from build123d import *

# Parameters (mm, degrees)
BOSS_EXTRUDE1_DEPTH      = 15.06
BOSS_EXTRUDE2_DEPTH      = 3.175
SKETCH7_W                = 15.06
SKETCH7_H                = 28.575
BOSS_EXTRUDE3_DEPTH      = 25.4
BOSS_EXTRUDE3_DEPTH_BACK = 2.54
CUT_EXTRUDE1_START       = -0.254
CUT_EXTRUDE1_DEPTH       = 14.552
BOSS_EXTRUDE4_DEPTH      = 8.1
SKETCH8_R                = 5.1
CUT_EXTRUDE3_DEPTH       = 826.597233992
SKETCH15_R               = 6.096
CUT_EXTRUDE4_DEPTH       = 823.185140665
CUT_EXTRUDE6_DEPTH       = 0.254
SKETCH22_W               = 12.7
SKETCH22_H               = 3
CUT_EXTRUDE8_DEPTH       = 2.5
BOSS_EXTRUDE5_START      = -3.175
SKETCH23_R               = 1.13
BOSS_EXTRUDE5_DEPTH      = 11.377
CUT_EXTRUDE9_DEPTH       = 2
SKETCH25_W               = 12.7
SKETCH25_H               = 2.5
BOSS_EXTRUDE6_DEPTH      = 2
CUT_EXTRUDE11_DEPTH      = 826.590147754
BOSS_EXTRUDE7_DEPTH      = 19.886
FILLET1_R                = 2
SKETCH31_R               = 2
CUT_EXTRUDE12_DEPTH      = 826.405127723


with BuildPart() as part:
    # Sketch1 → Boss-Extrude1 (new body)
    with BuildSketch(Plane.XY):
        with BuildLine():
            ThreePointArc((768.898502001, 253.220496825), (772.473384001, 257.975032047), (771.279316377, 263.802517698))
            Line((771.279316377, 263.802517698), (754.541770866, 286.976250421))
            ThreePointArc((754.541770866, 286.976250421), (750.425558167, 289.761469174), (745.483441324, 289.235986934))
            Line((745.483441324, 289.235986934), (736.959388492, 285.051606769))
            Line((736.959388492, 285.051606769), (732.179744734, 283.489883627))
            ThreePointArc((732.179744734, 283.489883627), (729.115297933, 279.264699802), (732.179762843, 275.03952911))
            Line((732.179762843, 275.03952911), (736.959413295, 273.477826454))
            ThreePointArc((736.959413295, 273.477826454), (738.543478356, 272.323947498), (739.148316802, 270.459847389))
            Line((739.148316802, 270.459847389), (741.478441562, 249.420712606))
            ThreePointArc((741.478441562, 249.420712606), (746.159744473, 243.429023652), (753.614349117, 244.926956583))
            ThreePointArc((753.614349117, 244.926956583), (754.705448313, 245.901255726), (755.838945539, 246.825885552))
            Line((755.838945539, 246.825885552), (768.898502001, 253.220496825))
        make_face()
    extrude(amount=BOSS_EXTRUDE1_DEPTH)

    # Sketch1<4> → Boss-Extrude2 (add)
    with BuildSketch(Plane.XY):
        with BuildLine():
            Line((767.984780823, 261.422994326), (751.247235317, 284.596727042))
            ThreePointArc((751.247235317, 284.596727042), (747.696485062, 285.758701464), (745.498379419, 282.7377176))
            Line((745.498379419, 282.7377176), (745.498449109, 250.217566764))
            ThreePointArc((745.498449109, 250.217566764), (747.408500645, 247.30543855), (750.840510516, 247.897127523))
            ThreePointArc((750.840510516, 247.897127523), (758.022031433, 253.136086658), (766.249615232, 256.501766428))
            ThreePointArc((766.249615232, 256.501766428), (768.405251042, 258.508228422), (767.984780823, 261.422994326))
        make_face()
    extrude(amount=-BOSS_EXTRUDE2_DEPTH)

    # Sketch7 → Boss-Extrude3 (add, two sides)
    with BuildSketch(Plane(origin=(759.782778814, 84.147408332, 0), x_dir=(0, 0, 1), z_dir=(-0.9939228549686344, -0.11007887340901991, 0))) as boss_extrude3_sk:
        with Locations((7.53, 176.895767228)):
            Rectangle(SKETCH7_W, SKETCH7_H)
    extrude(amount=BOSS_EXTRUDE3_DEPTH)
    extrude(boss_extrude3_sk.sketch, amount=-BOSS_EXTRUDE3_DEPTH_BACK)

    # Sketch9 → Cut-Extrude1 (cut)
    with BuildSketch(Plane.XY.offset(15.06).offset(CUT_EXTRUDE1_START)):
        Polygon((731.533703152, 249.732332737), (729.101180207, 271.696039986), (716.478359949, 270.298038294), (718.910882894, 248.334331045), align=None)
    extrude(amount=-CUT_EXTRUDE1_DEPTH, mode=Mode.SUBTRACT)

    # Sketch11 → Boss-Extrude4 (add)
    with BuildSketch(Plane(origin=(0, 0, 0), x_dir=(-1, 0, 0), z_dir=(0, 0, -1))):
        with BuildLine():
            Line((-716.637403434, 242.971478152), (-713.491899626, 271.372823733))
            Line((-713.491899626, 271.372823733), (-735.830090144, 273.846821422))
            Line((-735.830090144, 273.846821422), (-736.959413295, 273.477826454))
            ThreePointArc((-736.959413295, 273.477826454), (-738.543478356, 272.323947498), (-739.148316802, 270.459847389))
            Line((-739.148316802, 270.459847389), (-739.148370366, 245.464611162))
            Line((-739.148370366, 245.464611162), (-716.637403434, 242.971478152))
        make_face()
    extrude(amount=BOSS_EXTRUDE4_DEPTH)

    # Sketch8 → Cut-Extrude3 (cut, through all)
    with BuildSketch(Plane.XY.offset(15.06)):
        with Locations((723.935575753, 257.835181621)):
            Circle(SKETCH8_R)
    extrude(amount=-CUT_EXTRUDE3_DEPTH, mode=Mode.SUBTRACT)

    # Sketch15 → Cut-Extrude4 (cut, through all)
    with BuildSketch(Plane(origin=(48.686517672, -99.431271016, 0), x_dir=(0.8981144857275971, 0.4397617201692911, 0), z_dir=(0.43976172016929105, -0.898114485727597, 0))):
        with Locations((794.095983967, 7.53212)):
            Circle(SKETCH15_R)
    extrude(amount=-CUT_EXTRUDE4_DEPTH, mode=Mode.SUBTRACT)

    # Sketch20 → Cut-Extrude6 (cut)
    with BuildSketch(Plane.XY.offset(15.06)):
        with BuildLine():
            Line((732.179762843, 275.03952911), (735.830090144, 273.846821422))
            Line((735.830090144, 273.846821422), (713.491899626, 271.372823733))
            Line((713.491899626, 271.372823733), (716.637403434, 242.971478152))
            Line((716.637403434, 242.971478152), (742.879500347, 245.877841005))
            ThreePointArc((742.879500347, 245.877841005), (748.034725116, 243.00680713), (753.614349117, 244.926956583))
            ThreePointArc((753.614349117, 244.926956583), (754.705448313, 245.901255726), (755.838945539, 246.825885552))
            Line((755.838945539, 246.825885552), (768.898502001, 253.220496825))
            ThreePointArc((768.898502001, 253.220496825), (772.473384001, 257.975032047), (771.279316377, 263.802517698))
            Line((771.279316377, 263.802517698), (754.541770866, 286.976250421))
            ThreePointArc((754.541770866, 286.976250421), (750.425558167, 289.761469174), (745.483441324, 289.235986934))
            Line((745.483441324, 289.235986934), (736.959388492, 285.051606769))
            Line((736.959388492, 285.051606769), (732.179744734, 283.489883627))
            ThreePointArc((732.179744734, 283.489883627), (729.115297933, 279.264699802), (732.179762843, 275.03952911))
        make_face()
        Polygon((718.910882894, 248.334331045), (731.533703152, 249.732332737), (729.101180207, 271.696039986), (716.478359949, 270.298038294), align=None, mode=Mode.SUBTRACT)
    extrude(amount=-CUT_EXTRUDE6_DEPTH, mode=Mode.SUBTRACT)


with BuildPart() as cut_extrude6_kept_piece:
    # of the separate pieces the step leaves, the one the design keeps (cut_extrude6_pieces_kept)
    add(part.part.solids().sort_by_distance((753.614349117, 244.926956583, 0))[0])

    # Sketch22 → Cut-Extrude8 (cut)
    with BuildSketch(Plane(origin=(-18.45893554, 166.669201308, 0), x_dir=(0.9939228549686345, 0.11007887340901987, 0), z_dir=(-0.11007887340901987, 0.9939228549686345, 0))):
        with Locations((748.228320584, -10.131)):
            Rectangle(SKETCH22_W, SKETCH22_H)
    extrude(amount=-CUT_EXTRUDE8_DEPTH, mode=Mode.SUBTRACT)

    # Sketch23 → Boss-Extrude5 (add)
    with BuildSketch(Plane.XY.offset(14.806).offset(BOSS_EXTRUDE5_START)):
        Polygon((716.94729595, 266.063926932), (729.570116208, 267.461928624), (729.101180207, 271.696039986), (716.478359949, 270.298038294), align=None)
        with Locations((723.024238078, 268.879983459)):
            Circle(SKETCH23_R, mode=Mode.SUBTRACT)
    extrude(amount=-BOSS_EXTRUDE5_DEPTH)

    # Sketch24 → Cut-Extrude9 (cut)
    with BuildSketch(Plane.XY.offset(0.254)):
        Polygon((716.94729595, 266.063926932), (717.27753257, 263.082158367), (729.900352828, 264.480160059), (729.570116208, 267.461928624), align=None)
    extrude(amount=-CUT_EXTRUDE9_DEPTH, mode=Mode.SUBTRACT)

    # Sketch25 → Boss-Extrude6 (add)
    with BuildSketch(Plane(origin=(-18.45893554, 166.669201308, 0), x_dir=(0.9939228549686345, 0.11007887340901987, 0), z_dir=(-0.11007887340901987, 0.9939228549686345, 0))):
        with Locations((748.228320584, -7.381)):
            Rectangle(SKETCH25_W, SKETCH25_H)
    extrude(amount=BOSS_EXTRUDE6_DEPTH)

    # Sketch29 → Cut-Extrude11 (cut, through all)
    with BuildSketch(Plane.XY.offset(14.806)):
        Polygon((752.228042412, 251.293092232), (766.597874183, 258.329279755), (760.309281585, 271.1723169), (745.939449813, 264.136129378), align=None)
    extrude(amount=-CUT_EXTRUDE11_DEPTH, mode=Mode.SUBTRACT)

    # Sketch30 → Boss-Extrude7 (add)
    with BuildSketch(Plane.XY.offset(14.806)):
        with BuildLine():
            Line((729.789433052, 273.177806997), (735.830090144, 273.846821422))
            Line((735.830090144, 273.846821422), (732.179762843, 275.03952911))
            ThreePointArc((732.179762843, 275.03952911), (730.271210596, 276.27473784), (729.223019165, 278.292064539))
            Line((729.223019165, 278.292064539), (729.789433052, 273.177806997))
        make_face()
    extrude(amount=-BOSS_EXTRUDE7_DEPTH)

    # Fillet1
    fillet1_edges = [cut_extrude6_kept_piece.edges().sort_by_distance(p)[0] for p in [
        (729.789433052, 273.177806997, 4.863),
    ]]
    fillet(fillet1_edges, radius=FILLET1_R)

    # Sketch31 → Cut-Extrude12 (cut, through all)
    with BuildSketch(Plane(origin=(0, 0, 0), x_dir=(-1, 0, 0), z_dir=(0, 0, -1))):
        with Locations((-733.560297933, 279.264709327)):
            Circle(SKETCH31_R)
    extrude(amount=-CUT_EXTRUDE12_DEPTH, mode=Mode.SUBTRACT)


solid = cut_extrude6_kept_piece.part
Geometry check sheet. Reference: the model listing, model coordinates, mm. A direction names the side the tool comes from. Coordinates: 2 decimals unless noted, no trailing zeros. Answer in a Markdown table with one row per item. Add a question column.
1) Material ranges on line 1 along Z through (x, y) = (731, 249); line 2 along X through (y, z) = (258.5, -2.5); line 3 along X through (y, z) = (252, 3), recorded low to high. Write a range as [from, to].
2) Cross-section at A-A, the plane z = -1. State how many separate pieces and enclosed holes the cut face has, then the cut area to 3 significant figures.
3) Set-up check for faces 4 (the flat face through (723, 265, -1.746)), 5 (the flat face through (725.134, 249.024, 3.234)), 6 (the cylindrical face through (730.293, 276.251, -2.504)): record each of +Z, -Z, +X, -X, +Y, -Y from which the full face is reachable in a straight line by a thin tool's end or side.
4) Gauge pin test, flat ends, axial feed: P1, Ø1.5, axis at y = 281.5, z = 1, coming from the +X side; P2, Ø3, axis at x = 725, y = 249.5, coming from the +Z side; P3, Ø1, axis at y = 261.5, z = -5.5, coming from the -X side; P4, Ø3, axis at y = 268.5, z = -5, coming from the -X side. Record the tip position at first contact, or that the pin passes through.
5) Release check for a two-part mould opening along X. For faces 1 (the flat face through (734.6, 284.28, 7.3)), 2 (the flat face through (766.63, 252.11, 4.01)), 3 (the flat face through (763.5, 264.66, 5.94)) record: +X half, -X half, draft (parallel to the pull), parting line (faces both ways), or undercut.
Check result:
| question | item | result |
|---|---|---|
| 1 | line 1 | z = [-8.1, 8.63], [11.63, 14.81] |
| 1 | line 2 | x = [714.92, 718.88], [728.99, 739.15], [745.5, 748.7], [766.51, 768.4] |
| 1 | line 3 | x = [715.64, 718.5], [731.28, 751.88], [753.67, 756.25], [765.33, 766.41] |
| 2 | separate pieces | 2 |
| 2 | enclosed holes | 3 |
| 2 | area | 895 mm² |
| 3 | face 4 | +Z |
| 3 | face 5 | none |
| 3 | face 6 | -Z, +Y |
| 4 | P1 | stops at x = 759.04 |
| 4 | P2 | stops at z = 14.81 |
| 4 | P3 | stops at x = 714.53 |
| 4 | P4 | stops at x = 713.64 |
| 5 | face 1 | -X half |
| 5 | face 2 | +X half |
| 5 | face 3 | undercut |
